Can you work these out from the model? Positions are in its coordinate system, mm. Coordinates: 2 decimals unless noted, no trailing zeros. Order: outer loops, then holes, each group sorted by start corner. A loop starts at its lowest first (then second) coordinate and runs counter-clockwise, first axis right, second up. Notation, with made-up numbers: (-15, 72) - (-1, 72) arc R21 cw to (-1, 90) - close; hole circle Ø7 at (-20, 6). An arc over 180 degrees is marked (long way). Return JSON: item names as keys, results as strings. Group by question number.
1) If I drill on line 1 along Y through (x, z) = (80, 9.25); line 2 along Y through (x, z) = (54, 2.75); line 3 along X through (y, z) = (-28.5, 9.25), over which ranges is the centre line in solid material (lowest first)?
2) Imagine slicing it at C-C (z = 12.75). Write out the boundary of the cut face in (x, y).
3) Imagine slicing it at B-B (y = -104). Write out the boundary of the cut face in (x, z), and give its area (3 significant figures).
4) If we mould it in two halves opening along Y, with no side actions, what happens to faces 1 (the face through (68.077, -113.692, 10.14)), 2 (the face through (114, -108, 0)), 3 (the face through (20.416, -76.192, 10.14))? For each: pulls with the +Y half, pulls with the -Y half, needs draft (parallel to the pull), parting line crosses it, or undercut.
5) Imagine slicing it at A-A (x = 80). Write out the boundary of the cut face in (y, z), and give its area (3 significant figures).
6) For pin 1 Ø8 at (y, z) = (-75.5, 5.5) entering from -X; pin 2 Ø1.5 at (y, z) = (-73, 16) entering from -X; pin 3 Ø1 at (x, z) = (77, 2.5) entering from +Y, each with a flat end and sliding along its axis, tell me the tip position at first contact or that it passes through.
7) Imagine slicing it at D-D (x = 144.5). Write out the boundary of the cut face in (y, z), and give its area (3 significant figures).
Autodesk Inventor part; units mm, degrees
ref_plane "YZ Plane" through (0, 0, 0) normal (1, 0, 0) x (0, 1, 0)
ref_plane "XZ Plane" through (0, 0, 0) normal (0, 1, 0) x (-1, 0, 0)
ref_plane "XY Plane" through (0, 0, 0) normal (0, 0, 1) x (1, 0, 0)
sketch "Sketch1" plane through (0, 0, 0) normal (0, 0, 1) x (1, 0, 0)
  line L0 (0, 0) -> (160, 0)
  line L1 (160, 0) -> (118.589, -154.5481)
  line L2 (0, 0) -> (41.411, -154.5481)
  line L3 (41.411, -154.5481) -> (118.589, -154.5481)
  dimension "d0" = 160
  dimension "d1" = 160
  dimension "d2" = 160
  dimension "d3" = 75
  dimension "d4" = 75
extrude "Extrusion1" add sketch "Sketch1" along normal blind 20
sketch "Sketch5" plane through (0, 0, 20) normal (0, 0, 1) x (1, 0, 0)
  line L0 (160, 0) -> (0, 0)
  line L1 (160, 0) -> (256.5926, -25.8819)
  line L2 (118.589, -154.5481) -> (41.411, -154.5481)
  line L3 (118.589, -154.5481) -> (215.1815, -180.43)
  circle A0 centre (235.8871, -103.156) radius 80 construction
  arc A1 (215.1815, -180.43) -> (256.5926, -25.8819) centre (235.8871, -103.156) ccw
  line L4 (160, 0) -> (118.589, -154.5481)
  line L5 (0, 0) -> (41.411, -154.5481)
  line L6 (0, 0) -> (-96.5926, -25.8819)
  line L7 (41.411, -154.5481) -> (118.589, -154.5481)
  line L8 (41.411, -154.5481) -> (-55.1815, -180.43)
  circle A2 centre (-75.8871, -103.156) radius 80 construction
  arc A3 (-96.5926, -25.8819) -> (-55.1815, -180.43) centre (-75.8871, -103.156) ccw
  point P0 (90, 0)
  dimension "d25" = 100
  dimension "d26" = 100
  dimension "d27" = 160
  dimension "d30" = 100
  dimension "d31" = 100
  dimension "d32" = 160
extrude "Extrusion5" add sketch "Sketch5" against normal blind 20 contours L1 A1 L3 L4 | L5 L8 A3 L6
sketch "Sketch8" plane through (0, 0, 20) normal (0, 0, 1) x (1, 0, 0)
  line L0 (41.411, -154.5481) -> (118.589, -154.5481)
  line L1 (0, 0) -> (41.411, -154.5481)
  line L2 (0, 0) -> (160, 0)
  line L3 (160, 0) -> (118.589, -154.5481)
  line L4 (0, 0) -> (160, 0)
  line L5 (0, 0) -> (-96.5926, -25.8819)
  arc A0 (-96.5926, -25.8819) -> (-55.1815, -180.43) centre (-75.8871, -103.156) ccw
  line L6 (-55.1815, -180.43) -> (41.411, -154.5481)
  line L7 (215.1815, -180.43) -> (118.589, -154.5481)
  arc A1 (215.1815, -180.43) -> (256.5926, -25.8819) centre (235.8871, -103.156) ccw
  line L8 (160, 0) -> (256.5926, -25.8819)
  line L9 (160, 0) -> (0, 0)
  line L10 (160, 0) -> (256.5926, -25.8819)
  line L11 (0, 0) -> (160, 0)
  point P0 (90, 0)
  point P1 (70, 0)
extrude "Extrusion7" cut sketch "Sketch8" against normal through all contours L6 A0 L5 L1 | L3 L8 A1 L7
sketch "Sketch9" plane through (0, 0, 20) normal (0, 0, 1) x (1, 0, 0)
  circle A0 centre (80, -304.672) radius 315
  line L0 (0, 0) -> (160, 0)
  dimension "d37" = 630
extrude "Extrusion8" add sketch "Sketch9" against normal blind 20 contours L0 A0 picked at (60.8492, 1.6815)
sketch "Sketch10" plane through (0, 0, 20) normal (0, 0, 1) x (1, 0, 0)
  circle A0 centre (80, -60) radius 55
  line L0 (41.411, -154.5481) -> (118.589, -154.5481)
  point P0 (0, 0)
  point P1 (80, -154.5481)
  dimension "d40" = 110
  dimension "d41" = 60
extrude "Extrusion9" cut sketch "Sketch10" against normal through all
properties part number "HA002" material "ABS Plastic"
Calculated:
{
 "1": {"line 1": "-154.55 to -115, -5 to 10.33", "line 2": "-154.55 to -108.47, -11.53 to 9.25", "line 3": "7.64 to 34.91, 125.09 to 152.36"},
 "2": {"outline": "(0, 0) - (41.41, -154.55) - (118.59, -154.55) - (160, 0) arc R315 ccw to start; hole circle Ø110 at (80, -60)"},
 "3": {"outline": "(27.87, 0) - (47, 0) - (47, 20) - (27.87, 20) - close; (113, 0) - (132.13, 0) - (132.13, 20) - (113, 20) - close", "area": "765 mm2"},
 "4": {"face 1": "undercut", "face 2": "needs draft", "face 3": "pulls with the -Y half"},
 "5": {"outline": "(-154.55, 0) - (-115, 0) - (-115, 20) - (-154.55, 20) - close; (-5, 0) - (10.33, 0) - (10.33, 20) - (-5, 20) - close", "area": "1,100 mm2"},
 "6": {"pin 1": "x = 19.16", "pin 2": "x = 19.36", "pin 3": "y = 10.32"},
 "7": {"outline": "(-57.85, 0) - (3.65, 0) - (3.65, 20) - (-57.85, 20) - close", "area": "1,230 mm2"}
}
